from build123d import *

# Parameters (mm, degrees)
SKETCH1_R                = 19
BOSS_EXTRUDE1_DEPTH      = 29
SPLIT1_SURFACE_1_BACK    = 62.066
SPLIT1_SURFACE_1_DEPTH   = 124.132
SPLIT1_SURFACE_2_BACK    = 62.066
SPLIT1_SURFACE_2_DEPTH   = 124.132
BODY_DELETE_KEEP_1_DEPTH = 29


# Read off the part's stored shape, not the designer's step: Body-Delete/Keep 1
with BuildPart() as part:
    # Sketch1 → Boss-Extrude1 (new body)
    with BuildSketch(Plane(origin=(0, 0, 0), x_dir=(1, 0, 0), z_dir=(0, 1, 0))):
        with Locations(Location((0, 0, 0), (0, 0, 270))):
            Circle(SKETCH1_R)
    extrude(amount=BOSS_EXTRUDE1_DEPTH)


with BuildPart() as body_2:
    # Split1: the piece behind the surface
    add(part.part)
    # Split1 surface: a surface, the sketch's curves swept straight by 124.132 mm
    with BuildLine(Plane.XY.offset(-SPLIT1_SURFACE_1_BACK), mode=Mode.PRIVATE) as split1_surface_1_path:
        Line((0, 30.065054412), (0, -0.518911578))
    split1_surface_1 = Shell.extrude(split1_surface_1_path.wire(), (0 * SPLIT1_SURFACE_1_DEPTH, 0 * SPLIT1_SURFACE_1_DEPTH, 1 * SPLIT1_SURFACE_1_DEPTH))
    split(bisect_by=split1_surface_1, keep=Keep.BOTTOM)

    # Body-Delete/Keep 1 outline → Body-Delete/Keep 1 (cut)
    with BuildSketch(Plane(origin=(0, 0, 0), x_dir=(1, 0, 0), z_dir=(0, 1, 0))):
        with BuildLine():
            ThreePointArc((0, 19), (-19, 0), (0, -19))
            Line((0, -19), (0, 19))
        make_face()
    extrude(amount=BODY_DELETE_KEEP_1_DEPTH, mode=Mode.SUBTRACT)


with BuildPart() as part_1:
    add(part.part)

    # Split1: split by a surface, the side it looks to stays
    # Split1 surface: a surface, the sketch's curves swept straight by 124.132 mm
    with BuildLine(Plane.XY.offset(-SPLIT1_SURFACE_2_BACK), mode=Mode.PRIVATE) as split1_surface_2_path:
        Line((0, 30.065054412), (0, -0.518911578))
    split1_surface_2 = Shell.extrude(split1_surface_2_path.wire(), (0 * SPLIT1_SURFACE_2_DEPTH, 0 * SPLIT1_SURFACE_2_DEPTH, 1 * SPLIT1_SURFACE_2_DEPTH))
    split(bisect_by=split1_surface_2, keep=Keep.TOP)


solid = part_1.part
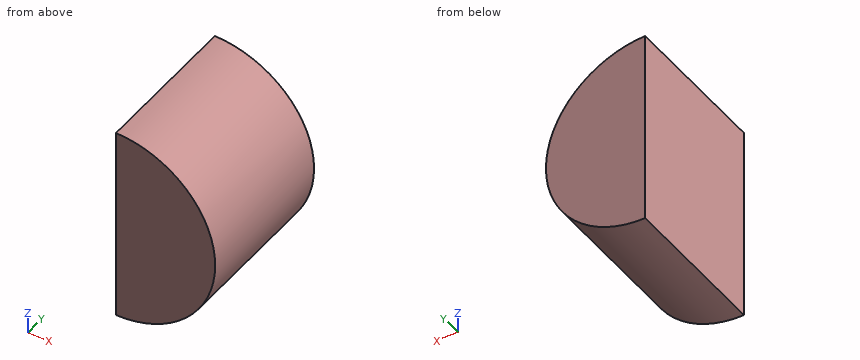
Model file for the job. Use its own axes, mm. Give positions to 0.01 mm unless a question says otherwise; leave off trailing zeros. Loops run counter-clockwise (first coordinate to the right, second up) from the corner with the lowest first, then second, coordinate; pieces in that order, holes last.
1) Saw through at B-B (z = -17). Write the cut outline in (x, y).
2) Wall check: line 1 (Z direction, x = 14.25, y = 18.25); line 2 (Z direction, x = 8.5, y = 10); line 3 (X direction, y = 4, z = 3.5). Give the ranges that are in metal, low to high.
3) Saw through at A-A (y = 25.25). Write the cut outline in (x, z), plus the area to 3 significant figures.
4) Saw through at C-C (x = 15). Write the cut outline in (y, z), plus the area to 3 significant figures.
5) Flat gauge pins, fed straight in: pin 1 Ø3 at (x, y) = (13, 25) entering from -Z; pin 2 Ø6 at (x, y) = (4, 7.5) entering from +Z; pin 3 Ø5 at (x, y) = (3, 10) entering from -Z. Where does each tip first touch, or does it go through?
Answer block:
1. outline: (0, 0) - (8.49, 0) - (8.49, 29) - (0, 29) - close
2. line 1: z = -12.57 to 12.57
2. line 2: z = -16.99 to 16.99
2. line 3: x = 0 to 18.67
3. outline: (0, -19) arc R19 ccw to (0, 19) - close
3. area: 567 mm2
4. outline: (0, -11.66) - (29, -11.66) - (29, 11.66) - (0, 11.66) - close
4. area: 676 mm2
5. pin 1: stops at z = -15.12
5. pin 2: stops at z = 18.97
5. pin 3: stops at z = -18.99
